Part model, mm, in its own coordinate system. A direction names the side the tool comes from. Give positions to 0.01 mm unless a question says otherwise; leave off trailing zeros. Order: outer loops, then holes, each group sorted by start corner. A loop starts at its lowest first (then second) coordinate and runs counter-clockwise, first axis right, second up. Notation, with made-up numbers: (69.5, -11) - (98.5, -11) arc R23 ccw to (98.5, 6) - close; hole circle Ø6 at (-10.5, 45). An arc over 180 degrees is marked (long way). One line per item, written item: value.
```python
from build123d import *

# Parameters (mm, degrees)
SKETCH_1_R               = 16
EXTRUDE_1_DEPTH          = 11
SKETCH_2_R               = 13.2
CUT_EXTRUDE_1_DEPTH      = 9.35
SKETCH_3_R               = 2
CUT_EXTRUDE_3_DEPTH      = 9.35
PATTERN_CIRCULAR_3_COUNT = 3
SKETCH_4_R               = 3.4
EXTRUDE_2_DEPTH          = 17.75
SKETCH_5_R               = 1.5
CUT_EXTRUDE_4_DEPTH      = 25.75
SKETCH_6_R               = 18.6
SKETCH_6_R_2             = 16
EXTRUDE_4_DEPTH          = 2.95
EXTRUDE_4_DEPTH_BACK     = 13.95


with BuildPart() as part:
    # ｽｹｯﾁ1 → ﾎﾞｽ - 押し出し1 (new body)
    with BuildSketch(Plane(origin=(0, 0, 0), x_dir=(0, 0, -1), z_dir=(1, 0, 0))):
        Circle(SKETCH_1_R)
    extrude(amount=EXTRUDE_1_DEPTH)

    # ｽｹｯﾁ2 → ｶｯﾄ - 押し出し1 (cut)
    with BuildSketch(Plane(origin=(11, 0, 0), x_dir=(0, 0, -1), z_dir=(1, 0, 0))):
        Circle(SKETCH_2_R)
    extrude(amount=-CUT_EXTRUDE_1_DEPTH, mode=Mode.SUBTRACT)

    # ｽｹｯﾁ3 → ｶｯﾄ - 押し出し3 (cut)
    with BuildSketch(Plane.ZY):
        with Locations((4.685675375, 6.484168897)):
            Circle(SKETCH_3_R)
    cut_extrude_3 = extrude(amount=-CUT_EXTRUDE_3_DEPTH, mode=Mode.SUBTRACT)

    # 円形ﾊﾟﾀｰﾝ3: ｶｯﾄ - 押し出し3 ×3 about axis
    pattern_circular_3_axis = Axis((0, 0, 0), (1, 0, 0))
    for i in range(1, PATTERN_CIRCULAR_3_COUNT):
        add(cut_extrude_3.rotate(pattern_circular_3_axis, i * 360 / PATTERN_CIRCULAR_3_COUNT), mode=Mode.SUBTRACT)

    # ｽｹｯﾁ4 → ﾎﾞｽ - 押し出し2 (add)
    with BuildSketch(Plane(origin=(1.65, 0, 0), x_dir=(0, 0, -1), z_dir=(1, 0, 0))):
        Circle(SKETCH_4_R)
    extrude(amount=EXTRUDE_2_DEPTH)

    # ｽｹｯﾁ5 → ｶｯﾄ - 押し出し4 (cut)
    with BuildSketch(Plane(origin=(19.4, 0, 0), x_dir=(0, 0, -1), z_dir=(1, 0, 0))):
        Circle(SKETCH_5_R)
    extrude(amount=-CUT_EXTRUDE_4_DEPTH, mode=Mode.SUBTRACT)

    # ｽｹｯﾁ6 → ﾎﾞｽ - 押し出し4 (add, two sides)
    with BuildSketch(Plane.ZY) as extrude_4_sk:
        Circle(SKETCH_6_R)
        Circle(SKETCH_6_R_2, mode=Mode.SUBTRACT)
    extrude(amount=EXTRUDE_4_DEPTH)
    extrude(extrude_4_sk.sketch, amount=-EXTRUDE_4_DEPTH_BACK)


solid = part.part
```
1) Slice it at C-C on y = 11.5. Write the cut outline in (x, z).
Answer:
outline: (-2.95, -14.62) - (13.95, -14.62) - (13.95, -11.12) - (11, -11.12) - (11, -6.48) - (1.65, -6.48) - (1.65, 6.48) - (11, 6.48) - (11, 11.12) - (13.95, 11.12) - (13.95, 14.62) - (-2.95, 14.62) - (-2.95, 11.12) - (0, 11.12) - (0, -11.12) - (-2.95, -11.12) - close
2) Slice it at D-D on x = 17.25. Write the cut outline in (y, z).
Answer:
outline: circle Ø6.8 at (0, 0); hole circle Ø3 at (0, 0)
3) Slice it at A-A on x = 3.5. Write the cut outline in (y, z), then the cut area to 3 significant figures.
Answer:
outline: circle Ø37.2 at (0, 0); circle Ø6.8 at (0, 0); hole circle Ø26.4 at (0, 0); hole circle Ø3 at (0, 0)
area: 569 mm2
4) Wall check: line 1 along Y through (x, z) = (-0.65, 0); line 2 along Z through (x, y) = (2, -2); line 3 along X through (y, z) = (-12, -3). Give the ranges that are in metal, low to high. Write a range as [from, to].
Answer:
line 1: y = [-18.6, -16], [16, 18.6]
line 2: z = [-18.49, -13.05], [-2.75, 2.75], [13.05, 18.49]
line 3: x = [0, 1.65]
5) Which spindle directions (+Z, -Z, +X, -X, +Y, -Y) get a long thin tool onto all of the face, cutting with end or side? Do faces 4 (the face through (-1.45, -15.62, -3.47)), 5 (the face through (10.4, -3.32, 0.74)), 6 (the face through (0.813, 5.718, 6.533)). Say none if no direction does.
Answer:
face 4: -X
face 5: +X
face 6: +X, -X
6) Drop flat-ended pins along their axis: P1, Ø4, axis at x = 2.5, y = -7, coming from the -Z side; P2, Ø19, axis at y = 0, z = 0, coming from the -X side; P3, Ø2, axis at x = 5.5, y = -13, coming from the -Z side. Give the stop position or say it passes through.
Answer:
P1: stops at z = -17.92
P2: stops at x = 0
P3: stops at z = -14.21
7) Slice it at B-B on z = 0. Write the cut outline in (x, y).
Answer:
outline: (-2.95, -18.6) - (13.95, -18.6) - (13.95, -16) - (11, -16) - (11, -13.2) - (1.65, -13.2) - (1.65, -3.4) - (19.4, -3.4) - (19.4, -1.5) - (0, -1.5) - (0, -16) - (-2.95, -16) - close; (-2.95, 16) - (0, 16) - (0, 1.5) - (19.4, 1.5) - (19.4, 3.4) - (1.65, 3.4) - (1.65, 13.2) - (11, 13.2) - (11, 16) - (13.95, 16) - (13.95, 18.6) - (-2.95, 18.6) - close
8) Two-plate mould, pull along Z, no slides. Class faces 1 (the face through (-2.95, 15.24, 5.42)), 2 (the face through (12.45, -15.62, -3.47)), 3 (the face through (5.382, 15.684, 9.999)): pulls with the +Z half, pulls with the -Z half, needs draft (parallel to the pull), parting line crosses it, or undercut.
Answer:
face 1: needs draft
face 2: undercut
face 3: parting line crosses it
